```python
from build123d import *

# Parameters (mm, degrees)
F0_W      = 304.8
F0_H      = 25.4
F1_DEPTH  = 96.8248
F2_W      = 19.05
F2_H      = 25.4
F3_DEPTH  = 71.4248
F4_W      = 34.925
F4_H      = 25.4
F4_W_2    = 171.45
F5_DEPTH  = 6.6548
F6_R      = 2.159
F7_DEPTH  = 96.8258
F8_R      = 3.937
F9_DEPTH  = 93.98
F10_R     = 3.970807
F10_R_2   = 4.064
F11_DEPTH = 25.401
F10_R_3   = 6.731
F12_DEPTH = 12.7


with BuildPart() as f1:
    # F0 (on Top) → F1 (new body)
    with BuildSketch(Plane.XY):
        Rectangle(F0_W, F0_H)
    extrude(amount=F1_DEPTH)

    # F2 (on face) → F3 (cut)
    with BuildSketch(Plane.XY.offset(96.8248)):
        with Locations((-142.875, 0)):
            Rectangle(F2_W, F2_H)
        with Locations((142.875, 0)):
            Rectangle(F2_W, F2_H)
    extrude(amount=-F3_DEPTH, mode=Mode.SUBTRACT)

    # F4 (on face) → F5 (cut)
    with BuildSketch(Plane.XY.offset(96.8248)):
        with Locations((-115.8875, 0)):
            Rectangle(F4_W, F4_H)
        Rectangle(F4_W_2, F4_H)
        with Locations((115.8875, 0)):
            Rectangle(F4_W, F4_H)
    extrude(amount=-F5_DEPTH, mode=Mode.SUBTRACT)

    # F6 (on face) → F7 (cut, through all)
    with BuildSketch(Plane(origin=(0, 0, 0), x_dir=(1, 0, 0), z_dir=(0, 0, -1))):
        with Locations((-92.075, 0)):
            Circle(F6_R)
        with Locations((92.075, 0)):
            Circle(F6_R)
    extrude(amount=-F7_DEPTH, mode=Mode.SUBTRACT)

    # F8 (on face) → F9 (cut)
    with BuildSketch(Plane(origin=(0, 0, 0), x_dir=(1, 0, 0), z_dir=(0, 0, -1))):
        with Locations((-92.075, 0)):
            Circle(F8_R)
        with Locations((92.075, 0)):
            Circle(F8_R)
    extrude(amount=-F9_DEPTH, mode=Mode.SUBTRACT)

    # F10 (on face) → F11 (cut, through all)
    with BuildSketch(Plane.XY.offset(25.4)):
        with Locations((142.875, 0)):
            Circle(F10_R)
        with Locations((-142.875, 0)):
            Circle(F10_R_2)
    extrude(amount=-F11_DEPTH, mode=Mode.SUBTRACT)

    # F10 (on face) → F12 (cut)
    with BuildSketch(Plane.XY.offset(25.4)):
        with Locations((-142.875, 0)):
            Circle(F10_R_3)
        with Locations((-142.875, 0)):
            Circle(F10_R_2, mode=Mode.SUBTRACT)
        with Locations((142.875, 0)):
            Circle(F10_R_3)
        with Locations((142.875, 0)):
            Circle(F10_R, mode=Mode.SUBTRACT)
    extrude(amount=-F12_DEPTH, mode=Mode.SUBTRACT)


solid = f1.part
```
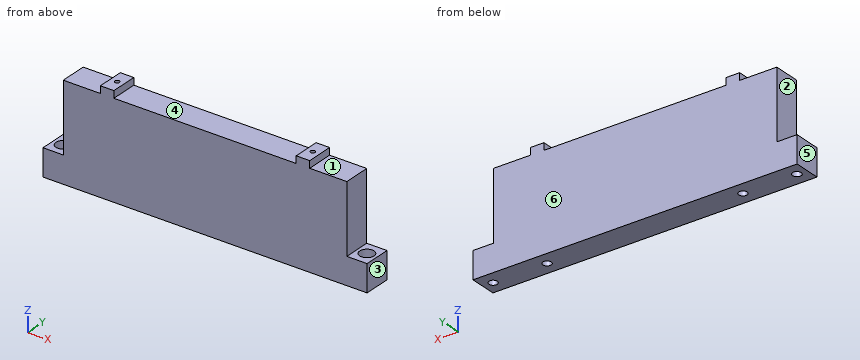
The listing builds one solid part. Answer for the finished solid, in the listing's coordinates (mm). Face numbers are marked on the shaded views. A direction names the side the tool comes from. Round coordinates to 2 decimals unless told otherwise and drop trailing zeros. Loops run counter-clockwise (first coordinate to the right, second up) from the corner with the lowest first, then second, coordinate; pieces in that order, holes last. Notation, with made-up numbers: (64, 65) - (97, 65) arc R19 cw to (97, 91) - close; hole circle Ø3 at (1.25, 89). An arc over 180 degrees is marked (long way). Return JSON: item names as keys, results as strings. Group by question number.
1. The mould has two halves that part along X. Classify the marked faces 4, 5 and 6: pulls with the +X half, pulls with the -X half, needs draft (parallel to the pull), parting line crosses it, or undercut.
2. The part is cut by section A-A on z = 7. Determine the outline of the cut face in (x, y) (3 decimals), then the cut area to 3 significant figures.
3. Consider probe 1 along X at (y, z) = (3.25, 50.5); probe 2 along X at (y, z) = (0, 95.05) (3 decimals); probe 3 along X at (y, z) = (-3.5, 46). Determine where each line is inside the solid, lowest interval first.
4. Each of these flat-tipped pins is pushed along its axis until it touches: P1, Ø1, axis at x = -2.5, y = -8.5, coming from the +Z side; P2, Ø6.5, axis at x = -145.5, y = -3, coming from the +Z side; P3, Ø12, axis at y = 1, z = 76, coming from the +X side. Where does it stop, or does it pass through?
5. The part is cut by section B-B on z = 76.5. Determine the outline of the cut face in (x, y) (3 decimals), then the cut area to 3 significant figures.
6. The part is cut by section C-C on x = -108. Determine the outline of the cut face in (y, z).
7. Which of the six approach directions +Z, -Z, +X, -X, +Y, -Y give full straight-line access (tool end or side, diameter ignored) to the marked faces 1, 2 and 3?
Resolved:
{
 "1": {"face 4": "undercut", "face 5": "pulls with the -X half", "face 6": "needs draft"},
 "2": {"outline": "(-152.4, -12.7) - (152.4, -12.7) - (152.4, 12.7) - (-152.4, 12.7) - close; hole circle Ø8.128 at (-142.875, 0); hole circle Ø7.874 at (-92.075, 0); hole circle Ø7.874 at (92.075, 0); hole circle Ø7.942 at (142.875, 0)", "area": "7,540 mm²"},
 "3": {"probe 1": "x = -133.35 to -94.3, -89.85 to 89.85, 94.3 to 133.35", "probe 2": "x = -98.425 to -94.234, -89.916 to -85.725, 85.725 to 89.916, 94.234 to 98.425", "probe 3": "x = -133.35 to -93.88, -90.27 to 90.27, 93.88 to 133.35"},
 "4": {"P1": "stops at z = 90.17", "P2": "stops at z = 25.4", "P3": "stops at x = 133.35"},
 "5": {"outline": "(-133.35, -12.7) - (133.35, -12.7) - (133.35, 12.7) - (-133.35, 12.7) - close; hole circle Ø7.874 at (-92.075, 0); hole circle Ø7.874 at (92.075, 0)", "area": "6,680 mm²"},
 "6": {"outline": "(-12.7, 0) - (12.7, 0) - (12.7, 90.17) - (-12.7, 90.17) - close"},
 "7": {"face 1": "+Z, +X, +Y, -Y", "face 2": "+Z, -X, +Y, -Y", "face 3": "+Z, -Z, +X, +Y, -Y"}
}
